Part model, mm, in its own coordinate system. Give positions to 0.01 mm unless a question says otherwise; leave off trailing zeros. Write each loop counter-clockwise with the first axis right and the second up, starting at its lowest first coordinate (ties: lowest second). Pieces come first, ordered by that corner, then holes.
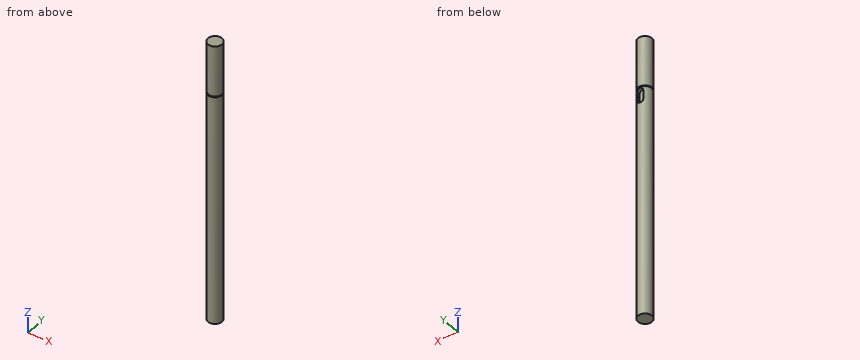
from build123d import *

# Parameters (mm, degrees)
CROQUIS1_R              = 5
SALIENTE_EXTRUIR1_DEPTH = 100
CORTAR_EXTRUIR1_START   = 2.5
CORTAR_EXTRUIR1_DEPTH   = 98.749688279


with BuildPart() as part:
    # Croquis1 → Saliente-Extruir1 (new, symmetric)
    with BuildSketch(Plane.XY):
        Circle(CROQUIS1_R)
    extrude(amount=SALIENTE_EXTRUIR1_DEPTH, both=True)

    # Croquis2 → Cortar-Extruir1 (cut, through all)
    with BuildSketch(Plane(origin=(0, 0, 0), x_dir=(1, 0, 0), z_dir=(0, 1, 0)).offset(CORTAR_EXTRUIR1_START)):
        with BuildLine():
            Line((2, -54.75), (2, -61.25))
            ThreePointArc((2, -61.25), (0, -63.25), (-2, -61.25))
            Line((-2, -61.25), (-2, -54.75))
            ThreePointArc((-2, -54.75), (0, -52.75), (2, -54.75))
        make_face()
    extrude(amount=CORTAR_EXTRUIR1_DEPTH, mode=Mode.SUBTRACT)

    # Croquis4 → Ranura para arandela de seguridad para ejes DIN 6799 - 91 (revolve, cut)
    with BuildSketch(Plane(origin=(0, 0, 100), x_dir=(0, 1, 0), z_dir=(-1, 0, 0))):
        with BuildLine():
            Line((4.65, 35.5), (6.641427447, 35.5))
            Line((6.641427447, 35.5), (6.641427447, 36.65))
            Line((6.641427447, 36.65), (4.65, 36.65))
            ThreePointArc((4.65, 36.65), (4.543933983, 36.606066017), (4.5, 36.5))
            Line((4.5, 36.5), (4.5, 35.65))
            ThreePointArc((4.5, 35.65), (4.543933983, 35.543933983), (4.65, 35.5))
        make_face()
    revolve(axis=Axis((0, 0, 150), (0, 0, -1)), mode=Mode.SUBTRACT)


solid = part.part
1) Flat gauge pins, fed straight in: P1, Ø4.5, axis at x = 0, z = 57, coming from the +Y side; P2, Ø0.6, axis at y = 4, z = 59, coming from the +X side; P3, Ø2, axis at y = 4, z = -17, coming from the +X side. Where does each tip first touch, or does it go through?
Check result:
P1: stops at y = 4.58
P2: stops at x = 3.36
P3: stops at x = 4
2) Drill centre lines: L1, parallel to Z at x = -4.5, y = -1; L2, parallel to X at y = -0.25, z = 17; L3, parallel to Y at x = -0.5, z = 42.5. Where is each one in solid material? Low to high.
Check result:
L1: z = -100 to 63.36, 64.49 to 100
L2: x = -4.99 to 4.99
L3: y = -4.97 to 4.97
3) Saw through at A-A (z = -40). Write the cut outline in (x, y).
Check result:
outline: circle Ø10 at (0, 0)
